Could you check a few things on this model? Use its own coordinates, in mm. A direction names the side the tool comes from. Round coordinates to 2 decimals unless told otherwise and drop trailing zeros. Loops run counter-clockwise (first coordinate to the right, second up) from the corner with the lowest first, then second, coordinate; pieces in that order, holes last. Notation, with made-up numbers: (45, -4) - (85, -4) arc R29 ccw to (85, 27) - close; hole circle Ø4 at (88, 46). An arc over 180 degrees is marked (long way). Use one line per item in the form item = value.
```python
from build123d import *

# Parameters (mm, degrees)
F0_W     = 140
F0_H     = 23.5
F1_DEPTH = 50
F2_W     = 16
F2_H     = 16
F3_DEPTH = 15
F4_R     = 11.74999
F5_R     = 5
F6_DEPTH = 140
F8_DEPTH = 25


# Not quite as in the source:
# - a fillet or chamfer is up to 0.001 mm smaller than in the source, because OpenCascade refuses the exact size


with BuildPart() as f1:
    # F0 (on Front) → F1 (new body)
    with BuildSketch(Plane.XZ):
        with Locations((-8.7296748534, -19.8372076215)):
            Rectangle(F0_W, F0_H)
    extrude(amount=F1_DEPTH)

    # F2 (on face) → F3 (cut)
    with BuildSketch(Plane(origin=(0, 0, 0), x_dir=(-1, 0, 0), z_dir=(0, 1, 0))):
        with Locations((-41.2703251466, -21.5872076215)):
            Rectangle(F2_W, F2_H)
        with Locations((58.7296748534, -21.5872076215)):
            Rectangle(F2_W, F2_H)
    extrude(amount=-F3_DEPTH, mode=Mode.SUBTRACT)

    # F4 (radius 11.75 in the source; OpenCascade refuses exactly that, so slightly less here)
    f4_edges = [f1.edges().sort_by_distance(p)[0] for p in [
        (-8.729675, -50, -8.087208),
        (-8.729675, -50, -31.587208),
    ]]
    fillet(f4_edges, radius=F4_R)

    # F5 (on face) → F6 (cut, through all)
    with BuildSketch(Plane(origin=(-78.7296748534, 0, 0), x_dir=(0, -1, 0), z_dir=(-1, 0, 0))):
        with Locations((38.25, -19.8372076215)):
            Circle(F5_R)
    extrude(amount=-F6_DEPTH, mode=Mode.SUBTRACT)

    # F7 (on face) → F8 (cut)
    with BuildSketch(Plane(origin=(0, 0, -31.5872076215), x_dir=(1, 0, 0), z_dir=(0, 0, -1))):
        Polygon((31.2703251466, 51.5), (-8.7296748534, 51.5), (-48.7296748534, 51.5), (-48.7296748534, 26.5), (-8.7296748534, 26.5), (31.2703251466, 26.5), align=None)
    extrude(amount=-F8_DEPTH, mode=Mode.SUBTRACT)


solid = f1.part
```
1. We'd pull the mould along X, two halves only. Please class faces 1 (the face through (31.27, -33, -20)), 2 (the face through (-10, -15, -8.087)), 3 (the face through (-78.73, -25, -20)): +X half, -X half, draft (parallel to the pull), parting line (faces both ways), or undercut.
Solution:
face_1 = undercut
face_2 = draft
face_3 = -X half
2. Please list where these lines run through material, in increasing order: line 1 along X through (y, z) = (-3.5, -13.75); line 2 along Z through (x, y) = (49.5, -38.25); line 3 along X through (y, z) = (-46, -25.5).
Solution:
line_1 = -78.73 to -66.73, -50.73 to 33.27, 49.27 to 61.27
line_2 = -31.59 to -24.84, -14.84 to -8.09
line_3 = -78.73 to -48.73, 31.27 to 61.27
3. For P1, Ø10, axis at x = -12.5, z = -28, coming from the -Y side; P2, Ø9, axis at y = -38.25, z = -19.84, coming from the -X side; P3, Ø3, axis at x = -58, z = -20.5, coming from the +Y side, each with a flat end and sliding along its axis, tell me the tip position at first contact or that it passes through.
Solution:
P1 = -26.5
P2 = through
P3 = -15
4. On a 3-axis mill with a long thin cutter (end or side, diameter ignored), from which of +Z, -Z, +X, -X, +Y, -Y can I reach the whole of each face in a straight line? I mean faces 4 (the face through (-9, -26.5, -20)), 5 (the face through (-10, -15, -31.587)), 6 (the face through (-50.73, -7, -22)). Say none if no direction works.
Solution:
face_4 = +Z, -Z, -Y
face_5 = -Z, +X, -X, +Y, -Y
face_6 = +Y
5. If we section it at D-D, the plane y = -46: Write out the boundary of the cut face in (x, z).
Solution:
outline = (-78.73, -28.67) - (-48.73, -28.67) - (-48.73, -11.01) - (-78.73, -11.01) - close; (31.27, -28.67) - (61.27, -28.67) - (61.27, -11.01) - (31.27, -11.01) - close
6. If we section it at C-C, the plane y = -11: Write out the boundary of the cut face in (x, z), plus the area to 3 significant figures.
Solution:
outline = (-78.73, -31.59) - (61.27, -31.59) - (61.27, -8.09) - (-78.73, -8.09) - close; hole (-66.73, -29.59) - (-50.73, -29.59) - (-50.73, -13.59) - (-66.73, -13.59) - close; hole (33.27, -29.59) - (49.27, -29.59) - (49.27, -13.59) - (33.27, -13.59) - close
area = 2,780 mm^2
7. If we section it at B-B, the plane z = -16.75: Write out the boundary of the cut face in (x, y).
Solution:
outline = (-78.73, -49.59) - (-48.73, -49.59) - (-48.73, -42.18) - (-78.73, -42.18) - close; (-78.73, -34.32) - (-48.73, -34.32) - (-48.73, -26.5) - (31.27, -26.5) - (31.27, -34.32) - (61.27, -34.32) - (61.27, 0) - (49.27, 0) - (49.27, -15) - (33.27, -15) - (33.27, 0) - (-50.73, 0) - (-50.73, -15) - (-66.73, -15) - (-66.73, 0) - (-78.73, 0) - close; (31.27, -49.59) - (61.27, -49.59) - (61.27, -42.18) - (31.27, -42.18) - close
